For this review, take the finished solid that the model builds, in its own axes (mm). A direction names the side the tool comes from. Give positions to 0.01 mm unless a question says otherwise; leave off trailing zeros. Loops run counter-clockwise (first coordinate to the right, second up) from the corner with the lowest first, then second, coordinate; pieces in that order, holes last.
```python
from build123d import *

# Parameters (mm, degrees)
SKETCH1_W                                        = 101.6
SKETCH1_H                                        = 50.8
BOSS_EXTRUDE1_DEPTH                              = 6.35
F_1_4_CLEARANCE_HOLE1_D                          = 6.7564
CBORE_FOR_1_4_SOCKET_HEAD_CAP_SCREW1_D           = 6.7564
CBORE_FOR_1_4_SOCKET_HEAD_CAP_SCREW1_CBORE_D     = 11.1125
CBORE_FOR_1_4_SOCKET_HEAD_CAP_SCREW1_CBORE_DEPTH = 6.35


with BuildPart() as part:
    # Sketch1 → Boss-Extrude1 (new, symmetric)
    with BuildSketch(Plane(origin=(0, 0, 0), x_dir=(1, 0, 0), z_dir=(0, 1, 0))):
        Rectangle(SKETCH1_W, SKETCH1_H)
    extrude(amount=BOSS_EXTRUDE1_DEPTH, both=True)

    # 1/4 Clearance Hole1 (through all)
    with Locations(Plane(origin=(0, 6.35, 0), x_dir=(1, 0, 0), z_dir=(0, 1, 0))):
        with Locations((-38.1, 12.7), (-38.1, -12.7), (38.1, 12.7), (38.1, -12.7)):
            Hole(F_1_4_CLEARANCE_HOLE1_D / 2)

    # CBORE for 1/4 Socket Head Cap Screw1 (through all)
    with Locations(Plane(origin=(0, 6.35, 0), x_dir=(1, 0, 0), z_dir=(0, 1, 0))):
        with Locations((0, 12.7), (0, -12.7)):
            CounterBoreHole(CBORE_FOR_1_4_SOCKET_HEAD_CAP_SCREW1_D / 2, CBORE_FOR_1_4_SOCKET_HEAD_CAP_SCREW1_CBORE_D / 2, CBORE_FOR_1_4_SOCKET_HEAD_CAP_SCREW1_CBORE_DEPTH)


solid = part.part
```
Q1. Consider section B-B on x = 38.1. Give the boundary of the cut face in (y, z).
Answers:
outline: (-6.35, -25.4) - (6.35, -25.4) - (6.35, -16.08) - (-6.35, -16.08) - close; (-6.35, -9.32) - (6.35, -9.32) - (6.35, 9.32) - (-6.35, 9.32) - close; (-6.35, 16.08) - (6.35, 16.08) - (6.35, 25.4) - (-6.35, 25.4) - close
Q2. For pin 1 Ø11 at (x, z) = (38.1, -12.7) entering from +Y; pin 2 Ø5.5 at (x, z) = (1.5, 15) entering from +Y, all flat-tipped, find the tip position at first contact; note any pin that passes through.
Answers:
pin 1: stops at y = 6.35
pin 2: stops at y = 0
Q3. Machinability: for faces 1 (the cylindrical face through (-41.322, -0.089, -13.715)), 2 (the flat face through (4, 0, -13)), which of the approach directions +Z, -Z, +X, -X, +Y, -Y give a long, thin tool a straight path to every point of the face, cutting with its end or side? Answer none if there is none.
Answers:
face 1: +Y, -Y
face 2: +Y
Q4. Consider section C-C on y = -1.75. Give the boundary of the cut face in (x, z), plus the area to 3 significant figures.
Answers:
outline: (-50.8, -25.4) - (50.8, -25.4) - (50.8, 25.4) - (-50.8, 25.4) - close; hole circle Ø6.76 at (-38.1, -12.7); hole circle Ø6.76 at (-38.1, 12.7); hole circle Ø6.76 at (0, -12.7); hole circle Ø6.76 at (0, 12.7); hole circle Ø6.76 at (38.1, -12.7); hole circle Ø6.76 at (38.1, 12.7)
area: 4,950 mm2
Q5. For probe 1 along Z at (x, y) = (-38.1, 1.5); probe 2 along X at (y, z) = (-4.5, 12.7); probe 3 along X at (y, z) = (1.75, 13), list the stretches that pass through material, from the lowest coordinate up.
Answers:
probe 1: z = -25.4 to -16.08, -9.32 to 9.32, 16.08 to 25.4
probe 2: x = -50.8 to -41.48, -34.72 to -3.38, 3.38 to 34.72, 41.48 to 50.8
probe 3: x = -50.8 to -41.46, -34.74 to -5.55, 5.55 to 34.74, 41.46 to 50.8
Q6. Mouldability with a two-part tool opening along X and no side actions: class faces 3 (the flat face through (-1, 0, -25.4)), 4 (the cylindrical face through (-41.221, -0.089, 13.994)), 5 (the flat face through (50.8, 0, 0)) as +X half, -X half, draft (parallel to the pull), parting line (faces both ways), or undercut.
Answers:
face 3: draft
face 4: undercut
face 5: +X half
Q7. Consider section A-A on z = 12.7. Give the boundary of the cut face in (x, y), plus the area to 3 significant figures.
Answers:
outline: (-50.8, -6.35) - (-41.48, -6.35) - (-41.48, 6.35) - (-50.8, 6.35) - close; (-34.72, -6.35) - (-3.38, -6.35) - (-3.38, 0) - (-5.56, 0) - (-5.56, 6.35) - (-34.72, 6.35) - close; (3.38, -6.35) - (34.72, -6.35) - (34.72, 6.35) - (5.56, 6.35) - (5.56, 0) - (3.38, 0) - close; (41.48, -6.35) - (50.8, -6.35) - (50.8, 6.35) - (41.48, 6.35) - close
area: 1,010 mm2
Q8. Consider section D-D on x = 0. Give the boundary of the cut face in (y, z), plus the area to 3 significant figures.
Answers:
outline: (-6.35, -25.4) - (6.35, -25.4) - (6.35, -18.26) - (0, -18.26) - (0, -16.08) - (-6.35, -16.08) - close; (-6.35, -9.32) - (0, -9.32) - (0, -7.14) - (6.35, -7.14) - (6.35, 7.14) - (0, 7.14) - (0, 9.32) - (-6.35, 9.32) - close; (-6.35, 16.08) - (0, 16.08) - (0, 18.26) - (6.35, 18.26) - (6.35, 25.4) - (-6.35, 25.4) - close
area: 418 mm2
